```python
from build123d import *

# Parameters (mm, degrees)
CHANFREIN1_SIZE = 2
CHANFREIN2_SIZE = 0.5


with BuildPart() as part:
    # Esquisse1 → Base-Révolution (revolve)
    with BuildSketch(Plane.XY, mode=Mode.PRIVATE) as base_r_volution_sk:
        Polygon((0, 6), (0, 9), (8, 9), (8, 10), (20, 10), (20, 4), (14, 4), (14, 6), align=None)
    revolve(base_r_volution_sk.sketch.rotate(Axis((0, 0, 0), (1, 0, 0)), 90), axis=Axis((0, 0, 0), (1, 0, 0)))

    # Chanfrein1
    chanfrein1_edges = [part.edges().sort_by_distance(p)[0] for p in [
        (20, 0, -10),
    ]]
    chamfer(chanfrein1_edges, length=CHANFREIN1_SIZE)

    # Chanfrein2
    chanfrein2_edges = [part.edges().sort_by_distance(p)[0] for p in [
        (0, 0, -9),
    ]]
    chamfer(chanfrein2_edges, length=CHANFREIN2_SIZE)


solid = part.part
```
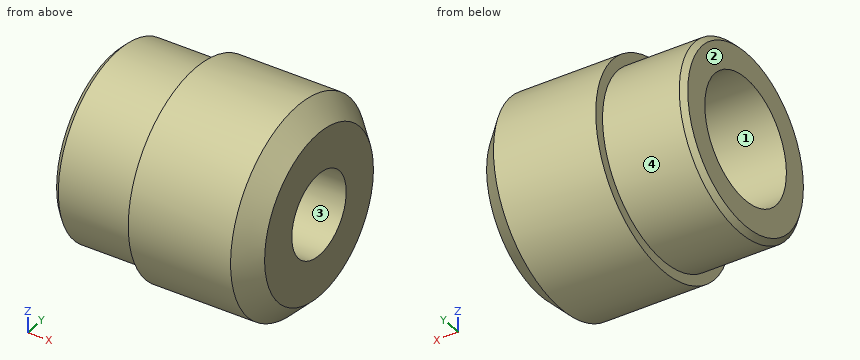
Here's how the part is built. I have some questions about the finished solid (model axes, mm). Face numbers are marked on the shaded views. Give positions to 0.01 mm unless a question says otherwise; leave off trailing zeros. Order: outer loops, then holes, each group sorted by start corner. A loop starts at its lowest first (then second) coordinate and runs counter-clockwise, first axis right, second up. Notation, with made-up numbers: M 41.5,17 L 90.5,17 A19 cw 90.5,54 Z; hole C 49.25,11 d7. An arc over 180 degrees is marked long. Use a Markdown table: item, result. Add a question column.
1. Suppose I cut it at C-C (x = 9.25). List the corners of the cut face in (y, z) for me.
2. Suppose I cut it at A-A (z = 0). List the corners of the cut face in (x, y) for me, and give its area (3 significant figures).
3. If we mould it in two halves opening along Z, with no side actions, what happens to the marked faces 1, 2, 3 and 4? For each: +Z half, -Z half, draft (parallel to the pull), parting line (faces both ways), or undercut.
4. For pin 1 Ø6 at (y, z) = (1.5, 6) entering from -X; pin 2 Ø7 at (y, z) = (0, 0) entering from +X; pin 3 Ø8 at (x, y) = (3, 7) entering from -Z; pin 4 Ø4 at (x, z) = (14, -4) entering from -Y, each with a flat end and sliding along its axis, tell me the tip position at first contact or that it passes through.
5. I need wall thicknesses on probe 1 along Y at (x, z) = (16.95, 0); probe 2 along Z at (x, y) = (10, 0.25); probe 3 along Y at (x, z) = (2.5, 0). Which ranges of each line are inside material? Lowest first, please. Write a range as from..to.
Results list:
| question | item | result |
|---|---|---|
| 1 | outline | C 0,0 d20; hole C 0,0 d12 |
| 2 | outline | M 0,-8.5 L 0.5,-9 L 8,-9 L 8,-10 L 18,-10 L 20,-8 L 20,-4 L 14,-4 L 14,-6 L 0,-6 Z; M 0,6 L 14,6 L 14,4 L 20,4 L 20,8 L 18,10 L 8,10 L 8,9 L 0.5,9 L 0,8.5 Z |
| 2 | area | 164 mm² |
| 3 | face 1 | undercut |
| 3 | face 2 | draft |
| 3 | face 3 | undercut |
| 3 | face 4 | parting line |
| 4 | pin 1 | stops at x = 0 |
| 4 | pin 2 | passes through |
| 4 | pin 3 | stops at z = -8.49 |
| 4 | pin 4 | stops at y = -9.8 |
| 5 | probe 1 | y = -10..-4, 4..10 |
| 5 | probe 2 | z = -10..-5.99, 5.99..10 |
| 5 | probe 3 | y = -9..-6, 6..9 |
